Source: CAD feature listing. Evaluate the final solid. Frame: model axes, mm. A direction names the side the tool comes from. Coordinates: 2 decimals unless noted, no trailing zeros. Order: outer loops, then holes, each group sorted by start corner. A loop starts at its lowest first (then second) coordinate and runs counter-clockwise, first axis right, second up.
Item 1: Contact query for flat-ended pins moving along their axis: P1, Ø12, axis at x = -42, z = 29, coming from the +Y side (3 decimals); P2, Ø1, axis at x = -46, y = 0, coming from the +Z side; P3, Ø12, axis at y = 28, z = 6, coming from the +X side; P4, Ø19, axis at x = 11.5, y = -1.5, coming from the +Z side. Output: stop coordinate, or through.
Item 2: Mould query, pull axis Z, two halves, no side actions, for faces 1 (the flat face through (-18.3, 26, 7.239)), 2 (the cylindrical face through (-47.812, 3.659, 33.464)), 3 (the cylindrical face through (-43.17, -3.26, 30.51)), 4 (the cylindrical face through (-5.506, -24.796, 4.829)). Classes: released by +Z, released by -Z, zero draft, split by the parting line, or undercut.
Item 3: Section D-D on y = -36.5. Return the cut outline in (x, z) (3 decimals).
Item 4: Ray query, line 1 (Y direction, x = 0, z = 7.95) (3 decimals); line 2 (Y direction, x = 0, z = 10.7); line 3 (Z direction, x = 20, y = -39). Return the intervals inside material, ascending.
Item 5: Section C-C on z = 11. Return the cut outline in (x, y), then the cut area to 3 significant figures.
Item 6: Section A-A on y = 0. Return the cut outline in (x, z) (1 decimal).
Item 7: Reachability of faces 5 (the flat face through (-46, 1.651, 30)), 6 (the cylindrical face through (-27.715, -21.251, 8.398)), 7 (the flat face through (10.6, 23.3, 0)) from +Z, -Z, +X, -X, +Y, -Y: full face, straight path, thin tool, end or side. Return the list, or none.
Item 8: Section B-B on x = 0. Return the cut outline in (y, z) (1 decimal).
from build123d import *

# Parameters (mm, degrees)
F0_R           = 50.8
F1_DEPTH       = 12.7
F2_R           = 38.1635
F3_DEPTH       = 3.175
F4_R           = 34.925
F4_R_2         = 31.623
F5_DEPTH       = 2.286
F4_R_3         = 25.4
F6_DEPTH       = 9.526
F8_R           = 5.715
F9_DEPTH       = 25.4
F10_R          = 3.175
F11_DEPTH      = 50.801
F11_DEPTH_BACK = 25.4
F13_W          = 3.302
F13_H          = 15.8052066865
F14_DEPTH      = 50.801


# Not quite as in the source:
# - a fillet or chamfer that OpenCascade refuses, or shapes differently, is made with other operations: its cross-section is extruded or revolved along the edge and cut away or added


with BuildPart() as f1:
    # F0 (on Top) → F1 (new body)
    with BuildSketch(Plane.XY):
        Circle(F0_R)
    extrude(amount=F1_DEPTH)

    # F2 (on face) → F3 (cut)
    with BuildSketch(Plane.XY.offset(12.7)):
        Circle(F2_R)
    extrude(amount=-F3_DEPTH, mode=Mode.SUBTRACT)

    # F4 (on face) → F5 (cut)
    with BuildSketch(Plane.XY.offset(9.525)):
        Circle(F4_R)
        Circle(F4_R_2, mode=Mode.SUBTRACT)
    extrude(amount=-F5_DEPTH, mode=Mode.SUBTRACT)

    # F4 (on face) → F6 (cut, through all)
    with BuildSketch(Plane.XY.offset(9.525)):
        Circle(F4_R_3)
    extrude(amount=-F6_DEPTH, mode=Mode.SUBTRACT)

    # F8 (on offset) → F9 (join)
    with BuildSketch(Plane.XY.offset(12.7)):
        with Locations((-44.45, 0)):
            Circle(F8_R)
    extrude(amount=F9_DEPTH)

    # F10 (on Front) → F11 (cut, two sides)
    with BuildSketch(Plane.XZ) as f11_sk:
        with Locations((-44.6398891509, 33.3248)):
            Circle(F10_R)
    extrude(amount=F11_DEPTH, mode=Mode.SUBTRACT)
    extrude(f11_sk.sketch, amount=-F11_DEPTH_BACK, mode=Mode.SUBTRACT)

    # F12: fillet of radius 2.54 on 1 edges, made by hand

    # F12_s1 → F12_t2 (revolve, cut)
    with BuildSketch(Plane.XZ):
        with BuildLine():
            ThreePointArc((-38.735, 35.56), (-39.4789487758, 37.3560512242), (-41.275, 38.1))
            Line((-41.275, 38.1), (-38.735, 38.1))
            Line((-38.735, 38.1), (-38.735, 35.56))
        make_face()
    revolve(axis=Axis((-44.45, 0, 38.1), (0, 0, 1)), mode=Mode.SUBTRACT)

    # F13 (on Right) → F14 (cut, through all)
    with BuildSketch(Plane.YZ):
        with Locations((0, 33.3026033432)):
            Rectangle(F13_W, F13_H)
    extrude(amount=-F14_DEPTH, mode=Mode.SUBTRACT)


solid = f1.part
Answer list:
1. P1: stops at y = 5.715
1. P2: stops at z = 25.4
1. P3: stops at x = 45.79
1. P4: passes through
2. face 1: released by +Z
2. face 2: undercut
2. face 3: undercut
2. face 4: zero draft
3. outline: (-35.333, 0) - (35.333, 0) - (35.333, 12.7) - (11.145, 12.7) - (11.145, 9.525) - (-11.145, 9.525) - (-11.145, 12.7) - (-35.333, 12.7) - close
4. line 1: y = -50.8 to -34.925, -31.623 to -25.4, 25.4 to 31.623, 34.925 to 50.8
4. line 2: y = -50.8 to -38.16, 38.16 to 50.8
4. line 3: z = 0 to 12.7
5. outline: circle Ø101.6 at (0, 0); hole circle Ø76.33 at (0, 0)
5. area: 3,530 mm2
6. outline: (-50.8, 0) - (-25.4, 0) - (-25.4, 9.5) - (-31.6, 9.5) - (-31.6, 7.2) - (-34.9, 7.2) - (-34.9, 9.5) - (-38.2, 9.5) - (-38.2, 12.7) - (-38.7, 12.7) - (-38.7, 25.4) - (-50.2, 25.4) - (-50.2, 12.7) - (-50.8, 12.7) - close; (25.4, 0) - (50.8, 0) - (50.8, 12.7) - (38.2, 12.7) - (38.2, 9.5) - (34.9, 9.5) - (34.9, 7.2) - (31.6, 7.2) - (31.6, 9.5) - (25.4, 9.5) - close
7. face 5: +Z, +X, -X
7. face 6: +Z
7. face 7: -Z, +X, -X, +Y, -Y
8. outline: (-50.8, 0) - (-25.4, 0) - (-25.4, 9.5) - (-31.6, 9.5) - (-31.6, 7.2) - (-34.9, 7.2) - (-34.9, 9.5) - (-38.2, 9.5) - (-38.2, 12.7) - (-50.8, 12.7) - close; (25.4, 0) - (50.8, 0) - (50.8, 12.7) - (38.2, 12.7) - (38.2, 9.5) - (34.9, 9.5) - (34.9, 7.2) - (31.6, 7.2) - (31.6, 9.5) - (25.4, 9.5) - close
